```python
from build123d import *

# Parameters (mm, degrees)
F0_W     = 153.123051
F0_H     = 89.177757
F0_R     = 10.398269
F0_R_2   = 10.580509
F0_R_3   = 11.411691
F0_R_4   = 10.35798
F1_DEPTH = 25.4
F3_DEPTH = 25.4


with BuildPart() as f1:
    # F0 (on Front) → F1 (new body)
    with BuildSketch(Plane.XZ):
        with Locations((0.864126, -0.691298)):
            Rectangle(F0_W, F0_H)
        with Locations((-59.451837, -30.762867)):
            Circle(F0_R, mode=Mode.SUBTRACT)
        with Locations((52.884482, -29.725916)):
            Circle(F0_R_2, mode=Mode.SUBTRACT)
        with Locations((-57.032287, 20.393362)):
            Circle(F0_R_3, mode=Mode.SUBTRACT)
        with Locations((51.15623, 22.121616)):
            Circle(F0_R_4, mode=Mode.SUBTRACT)
    extrude(amount=F1_DEPTH)

    # F2 (on face) → F3 (join)
    with BuildSketch(Plane.XZ.offset(25.4)):
        Polygon((17.54057, 9.526291), (0.520275, 19.953725), (-17.020295, 10.427433), (-17.54057, -9.526291), (-0.520275, -19.953725), (17.020295, -10.427433), align=None)
    extrude(amount=F3_DEPTH)


solid = f1.part
```
Source: CAD feature listing. Evaluate the final solid. Frame: model axes, mm. A direction names the side the tool comes from. Give positions to 0.01 mm unless a question says otherwise; leave off trailing zeros. Loops run counter-clockwise (first coordinate to the right, second up) from the corner with the lowest first, then second, coordinate; pieces in that order, holes last. Notation, with made-up numbers: (-33, 23) -> (-17, 23) arc R29 ccw to (-17, 60) -> close; hole circle Ø6 at (17.5, 9). An arc over 180 degrees is marked (long way). Put each result on its own line as item: value. Start each with the question number.
1) Draft query along X for faces 4 (the face through (-46.5, -12.5, 16)), 5 (the face through (9.15, -37.922, 14.667)), 6 (the face through (0, -50.8, 0)), 7 (the face through (-49.85, -12.52, -34.75)). Return one class per face: released by +X, released by -X, zero draft, split by the parting line, or undercut.
2) Reachability of faces 1 (the face through (8.127, -37.922, -15.257)), 2 (the face through (-8.127, -37.922, 15.257)), 3 (the face through (0, -25.4, 20)) from +Z, -Z, +X, -X, +Y, -Y: full face, straight path, thin tool, end or side. Return the list, or none.
3) Cut plane A-A (z = -36). Return loops of the section in (x, y).
4) Cut plane D-D (x = 15.5). Return loops of the section in (y, z), then the cut area to 3 significant figures.
5) Cut plane C-C (y = -43). Return loops of the section in (x, z), then the cut area to 3 significant figures.
6) Cut plane B-B (x = -55.5). Return loops of the section in (y, z).
7) Material intervals for probe 1 along X at (y, z) = (-21, -36); probe 2 along Z at (x, y) = (50, -11.5); probe 3 along X at (y, z) = (-24, -38), sorted ascending.
8) Contact query for a flat-ended pin moving along its axis: P1, Ø5, axis at x = 38, z = -11.5, coming from the -Y side. Output: stop coordinate, or through.
Results are:
1. face 4: undercut
1. face 5: released by +X
1. face 6: zero draft
1. face 7: undercut
2. face 1: -Z, +X, -Y
2. face 2: +Z, -X, -Y
2. face 3: -Y
3. outline: (-75.7, -25.4) -> (-68.43, -25.4) -> (-68.43, 0) -> (-75.7, 0) -> close; (-50.47, -25.4) -> (44.36, -25.4) -> (44.36, 0) -> (-50.47, 0) -> close; (61.4, -25.4) -> (77.43, -25.4) -> (77.43, 0) -> (61.4, 0) -> close
4. outline: (-50.8, -11.25) -> (-25.4, -11.25) -> (-25.4, -45.28) -> (0, -45.28) -> (0, 43.9) -> (-25.4, 43.9) -> (-25.4, 10.78) -> (-50.8, 10.78) -> close
4. area: 2,820 mm2
5. outline: (-17.54, -9.53) -> (-0.52, -19.95) -> (17.02, -10.43) -> (17.54, 9.53) -> (0.52, 19.95) -> (-17.02, 10.43) -> close
5. area: 1,040 mm2
6. outline: (-25.4, -45.28) -> (0, -45.28) -> (0, -40.38) -> (-25.4, -40.38) -> close; (-25.4, -21.14) -> (0, -21.14) -> (0, 9.09) -> (-25.4, 9.09) -> close; (-25.4, 31.7) -> (0, 31.7) -> (0, 43.9) -> (-25.4, 43.9) -> close
7. probe 1: x = -75.7 to -68.43, -50.47 to 44.36, 61.4 to 77.43
7. probe 2: z = -45.28 to -39.91, -19.55 to 11.83, 32.41 to 43.9
7. probe 3: x = -75.7 to -66.92, -51.99 to 46.29, 59.48 to 77.43
8. P1: stops at y = -25.4
